```python
from build123d import *

# Parameters (mm, degrees)
SKETCH_1_W          = 150
SKETCH_1_H          = 150
EXTRUDE_1_DEPTH     = 500
SKETCH_2_W          = 140
SKETCH_2_H          = 140
CUT_EXTRUDE_1_DEPTH = 501
MM_1_D              = 6


with BuildPart() as part:
    # 草图1 → 凸台-拉伸1 (new body)
    with BuildSketch(Plane.XY):
        Rectangle(SKETCH_1_W, SKETCH_1_H)
    extrude(amount=EXTRUDE_1_DEPTH)

    # 草图2 → 切除-拉伸1 (cut, through all)
    with BuildSketch(Plane.XY.offset(500)):
        Rectangle(SKETCH_2_W, SKETCH_2_H)
    extrude(amount=-CUT_EXTRUDE_1_DEPTH, mode=Mode.SUBTRACT)

    # 大小mm 暗销孔1 (through all)
    with Locations(Plane(origin=(0, 75, 0), x_dir=(1, 0, 0), z_dir=(0, 1, 0))):
        with Locations((-10, -50), (10, -50), (10, -70), (-10, -70)):
            Hole(MM_1_D / 2)


solid = part.part
```
The model under review builds one solid part; all positions refer to its coordinate system, in mm. A direction names the side the tool comes from. Coordinates: 2 decimals unless noted, no trailing zeros. Write each loop counter-clockwise with the first axis right and the second up, starting at its lowest first coordinate (ties: lowest second). Pieces come first, ordered by that corner, then holes.
1) To check wall thickness, follow probe 1 along X at (y, z) = (-72.8, 50); probe 2 along Z at (x, y) = (-10, 73); probe 3 along Y at (x, z) = (66, 430.5). State the ranges of each line that lie inside material, in increasing order.
2) Machinability: for faces 5 (the face through (-1, -75, 246)), 6 (the face through (70, -1, 254)), which of the approach directions +Z, -Z, +X, -X, +Y, -Y give a long, thin tool a straight path to every point of the face, cutting with its end or side? Answer none if there is none.
3) The part is to be moulded in two halves that separate along Y. For faces 1 (the face through (-75, -1, 246)), 2 (the face through (-1, 75, 246)), 3 (the face through (-1, 70, 254)), 4 (the face through (-70, -1, 254)), say which applies: pulls with the +Y half, pulls with the -Y half, needs draft (parallel to the pull), parting line crosses it, or undercut.
4) We need section C-C on z = 465.5. State the section outline as (x, y) points.
5) We need section A-A on y = -35. State the section outline as (x, z) points.
Answer list:
1. probe 1: x = -75 to -13, -7 to 7, 13 to 75
1. probe 2: z = 0 to 47, 53 to 67, 73 to 500
1. probe 3: y = -75 to -70, 70 to 75
2. face 5: +Z, -Z, +X, -X, -Y
2. face 6: +Z, -Z
3. face 1: needs draft
3. face 2: pulls with the +Y half
3. face 3: undercut
3. face 4: undercut
4. outline: (-75, -75) - (75, -75) - (75, 75) - (-75, 75) - close; hole (-70, -70) - (70, -70) - (70, 70) - (-70, 70) - close
5. outline: (-75, 0) - (-70, 0) - (-70, 500) - (-75, 500) - close; (70, 0) - (75, 0) - (75, 500) - (70, 500) - close
